CAD build for the part. Positions are in the model's coordinates, mm. Face numbers are marked on the shaded views. A direction names the side the tool comes from. Give positions to 0.01 mm unless a question says otherwise; leave off trailing zeros. Order: outer loops, then holes, each group sorted by start corner. A loop starts at its lowest first (then second) coordinate and runs counter-clockwise, first axis right, second up. Notation, with made-up numbers: (51.5, -31.5) -> (64.5, -31.5) arc R15 ccw to (64.5, -11.5) -> close; hole circle Ø1 at (9.25, 1.25). An arc over 180 degrees is marked (long way). Answer as CSV lines item,"result".
```python
from build123d import *

# Parameters (mm, degrees)
BODY_EXTRUD_DEPTH   = 154
BOSS_EXTRUDE2_DEPTH = 7
SKETCH3_R           = 27
BOSS_EXTRUDE3_DEPTH = 18
SKETCH4_R           = 14.5
BOSS_EXTRUDE4_DEPTH = 3
SKETCH5_R           = 7
BOSS_EXTRUDE5_DEPTH = 19
SKETCH6_R           = 9.5
BOSS_EXTRUDE6_DEPTH = 13
SKETCH7_R           = 1.5875
BOSS_EXTRUDE7_DEPTH = 30


with BuildPart() as part:
    # Body → Body_extrud (new body)
    with BuildSketch(Plane(origin=(0, 0, 0), x_dir=(1, 0, 0), z_dir=(0, 1, 0))):
        Polygon((-38.5, -35), (-38.5, -42), (-27, -42), (-27, -35), (38.5, -35), (38.5, 35), (-27, 35), (-27, 42), (-38.5, 42), (-38.5, 35), align=None)
    extrude(amount=BODY_EXTRUD_DEPTH)

    # Sketch2 → Boss-Extrude2 (add)
    with BuildSketch(Plane.XZ):
        with BuildLine():
            Line((-33.5, 22.426470588), (-22.120203818, 22.426470588))
            ThreePointArc((-22.120203818, 22.426470588), (0, 31.5), (22.120203818, 22.426470588))
            Line((22.120203818, 22.426470588), (33.5, 22.426470588))
            ThreePointArc((33.5, 22.426470588), (37.035533906, 20.962004494), (38.5, 17.426470588))
            Line((38.5, 17.426470588), (38.5, -17.426470588))
            ThreePointArc((38.5, -17.426470588), (37.035533906, -20.962004494), (33.5, -22.426470588))
            Line((33.5, -22.426470588), (22.120203818, -22.426470588))
            ThreePointArc((22.120203818, -22.426470588), (0, -31.5), (-22.120203818, -22.426470588))
            Line((-22.120203818, -22.426470588), (-33.5, -22.426470588))
            ThreePointArc((-33.5, -22.426470588), (-37.035533906, -20.962004494), (-38.5, -17.426470588))
            Line((-38.5, -17.426470588), (-38.5, 17.426470588))
            ThreePointArc((-38.5, 17.426470588), (-37.035533906, 20.962004494), (-33.5, 22.426470588))
        make_face()
    extrude(amount=BOSS_EXTRUDE2_DEPTH)

    # Sketch3 → Boss-Extrude3 (add)
    with BuildSketch(Plane(origin=(0, -7, 0), x_dir=(-1, 0, 0), z_dir=(0, -1, 0))):
        Circle(SKETCH3_R)
    extrude(amount=BOSS_EXTRUDE3_DEPTH)

    # Sketch4 → Boss-Extrude4 (add)
    with BuildSketch(Plane(origin=(0, -25, 0), x_dir=(-1, 0, 0), z_dir=(0, -1, 0))):
        Circle(SKETCH4_R)
    extrude(amount=BOSS_EXTRUDE4_DEPTH)

    # Sketch5 → Boss-Extrude5 (add)
    with BuildSketch(Plane(origin=(0, -28, 0), x_dir=(-1, 0, 0), z_dir=(0, -1, 0))):
        Circle(SKETCH5_R)
    extrude(amount=BOSS_EXTRUDE5_DEPTH)

    # Sketch6 → Boss-Extrude6 (add)
    with BuildSketch(Plane.XZ.offset(47)):
        Circle(SKETCH6_R)
    extrude(amount=BOSS_EXTRUDE6_DEPTH)

    # Sketch7 → Boss-Extrude7 (add)
    with BuildSketch(Plane.XZ.offset(60)):
        Circle(SKETCH7_R)
    extrude(amount=BOSS_EXTRUDE7_DEPTH)


solid = part.part
```
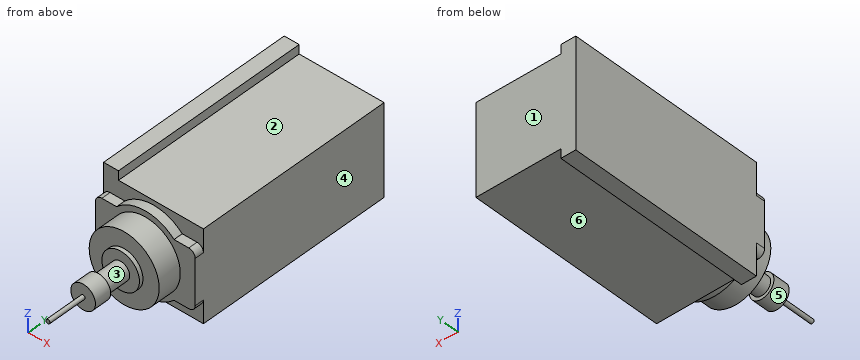
1) Band-saw the part on B-B, the plane y = -64.5. Write the cut outline in (x, z) (1 decimal), then the cut area to 3 significant figures.
Data:
outline,"circle Ø3.2 at (0, 0)"
area,"7.92 mm2"
2) Which spindle directions (+Z, -Z, +X, -X, +Y, -Y) get a long thin tool onto all of the face, cutting with end or side? Do the marked faces 4, 5 and 6. Say none if no direction does.
Data:
face 4,"+Z, -Z, +X, +Y, -Y"
face 5,"-Y"
face 6,"-Z, +X, +Y, -Y"
3) Band-saw the part on A-A, the plane y = 51. Write the cut outline in (x, z).
Data:
outline,"(-38.5, -42) -> (-27, -42) -> (-27, -35) -> (38.5, -35) -> (38.5, 35) -> (-27, 35) -> (-27, 42) -> (-38.5, 42) -> close"
4) Pin check, flat tips, straight feed: P1, Ø3.5, axis at y = 45, z = -40, coming from the +X side; P2, Ø19.5, axis at x = 8, y = 78, coming from the +Z side; P3, Ø19.5, axis at x = 21.5, y = 100.5, coming from the -Z side. Stop position of each tip, or through.
Data:
P1,"stops at x = -27"
P2,"stops at z = 35"
P3,"stops at z = -35"
5) Pull direction Y, two halves, no side cores. Call the marked faces 1, 2 and 3: pulls with the +Y half, pulls with the -Y half, needs draft (parallel to the pull), parting line crosses it, or undercut.
Data:
face 1,"pulls with the +Y half"
face 2,"needs draft"
face 3,"undercut"
6) Wall check: line 1 along Y through (x, z) = (-27, 30); line 2 along Z through (x, y) = (-21, 116); line 3 along Y through (x, z) = (-2.5, -13.5). Give the ranges that are in metal, low to high. Write a range as [from, to].
Data:
line 1,"y = [0, 154]"
line 2,"z = [-35, 35]"
line 3,"y = [-28, 154]"
